from build123d import *

# Parameters (mm, degrees)
TABAN_FLAN_1_DEPTH = 35


# Sheet-metal steps are written as plain solids
with BuildPart() as part:
    # Çizim1 → Taban-Flanş1 (new body)
    with BuildSketch(Plane.XY):
        with BuildLine():
            Line((619.494818874, -8.424828485), (98.926807278, -7.251557341))
            Line((98.926807278, -7.251557341), (43.504425744, -10.354452253))
            ThreePointArc((43.504425744, -10.354452253), (28.028820782, -11.029931963), (12.553215819, -10.354452253))
            ThreePointArc((12.553215819, -10.354452253), (5.187207724, -6.497959982), (0, 0))
            Line((0, 0), (2.280792838, 18.926510932))
            Line((2.280792838, 18.926510932), (60.45793545, 68.809534856))
            ThreePointArc((60.45793545, 68.809534856), (111.943036833, 92.83857175), (167.737234585, 103.567866957))
            ThreePointArc((167.737234585, 103.567866957), (406.337705204, 75.758628342), (635.459190458, 3.599891337))
            ThreePointArc((635.459190458, 3.599891337), (637.974703815, 2.109119279), (640, 0))
            ThreePointArc((640, 0), (632.566042161, -5.006768243), (623.989844607, -7.610667804))
            ThreePointArc((623.989844607, -7.610667804), (621.750134496, -8.060827589), (619.494818874, -8.424828485))
        make_face()
    extrude(amount=TABAN_FLAN_1_DEPTH)


solid = part.part
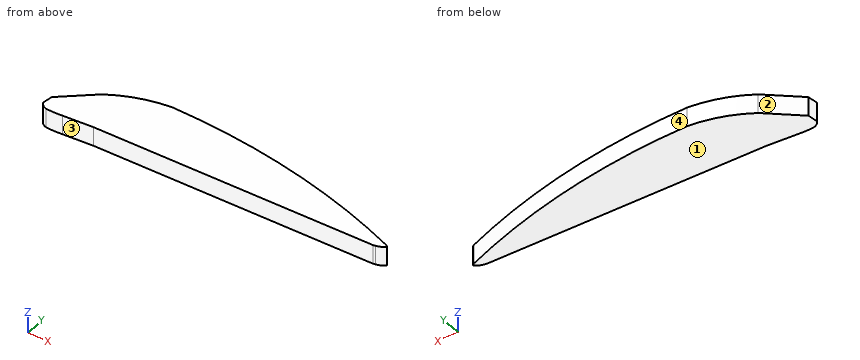
Geometry check sheet. Reference: the model listing, model coordinates, mm. Face numbers are marked on the shaded views. Give positions to 0.01 mm unless a question says otherwise; leave off trailing zeros. Order: outer loops, then holes, each group sorted by start corner. A loop starts at its lowest first (then second) coordinate and runs counter-clockwise, first axis right, second up.
1) Gauge pin test, flat ends, axial feed: pin 1 (4 mm diameter, centred on x = 153, z = 7.5, fed in from -Y); pin 2 (5 mm diameter, centred on x = 502.5, z = 12, fed in from +Y); pin 3 (1.5 mm diameter, centred on x = 411.5, z = 5.5, fed in from +Y). Record the tip position at first contact, or that the pin passes through.
Results are:
pin 1: stops at y = -7.38
pin 2: stops at y = 51.99
pin 3: stops at y = 74.81
2) Cross-section at B-B (x = 601). Record the boundary of the cut face in (y, z), then the cut area to 3 significant figures.
Results are:
outline: (-8.38, 0) - (17.56, 0) - (17.56, 35) - (-8.38, 35) - close
area: 908 mm2
3) Material ranges on probe 1 along X at (y, z) = (3.5, 4); probe 2 along Y at (x, z) = (159.5, 10); probe 3 along Y at (x, z) = (181, 12), recorded low to high.
Results are:
probe 1: x = 0.42 to 635.69
probe 2: y = -7.39 to 102.87
probe 3: y = -7.44 to 103.21
4) Draft check along X on the marked faces 1, 2, 3 and 4. Enter one of: released by +X, released by -X, zero draft, split by the parting line, or undercut.
Results are:
face 1: zero draft
face 2: released by -X
face 3: undercut
face 4: released by +X
5) Cross-section at A-A (z = 16.5). Record the boundary of the cut face in (x, y), then the cut area to 3 significant figures.
Results are:
outline: (0, 0) arc R20.19 ccw to (12.55, -10.35) arc R177.61 ccw to (43.5, -10.35) - (98.93, -7.25) - (619.49, -8.42) arc R59.6 ccw to (623.99, -7.61) arc R30.19 ccw to (640, 0) arc R10.84 ccw to (635.46, 3.6) arc R1272.37 ccw to (167.74, 103.57) arc R230.9 ccw to (60.46, 68.81) - (2.28, 18.93) - close
area: 49,800 mm2
